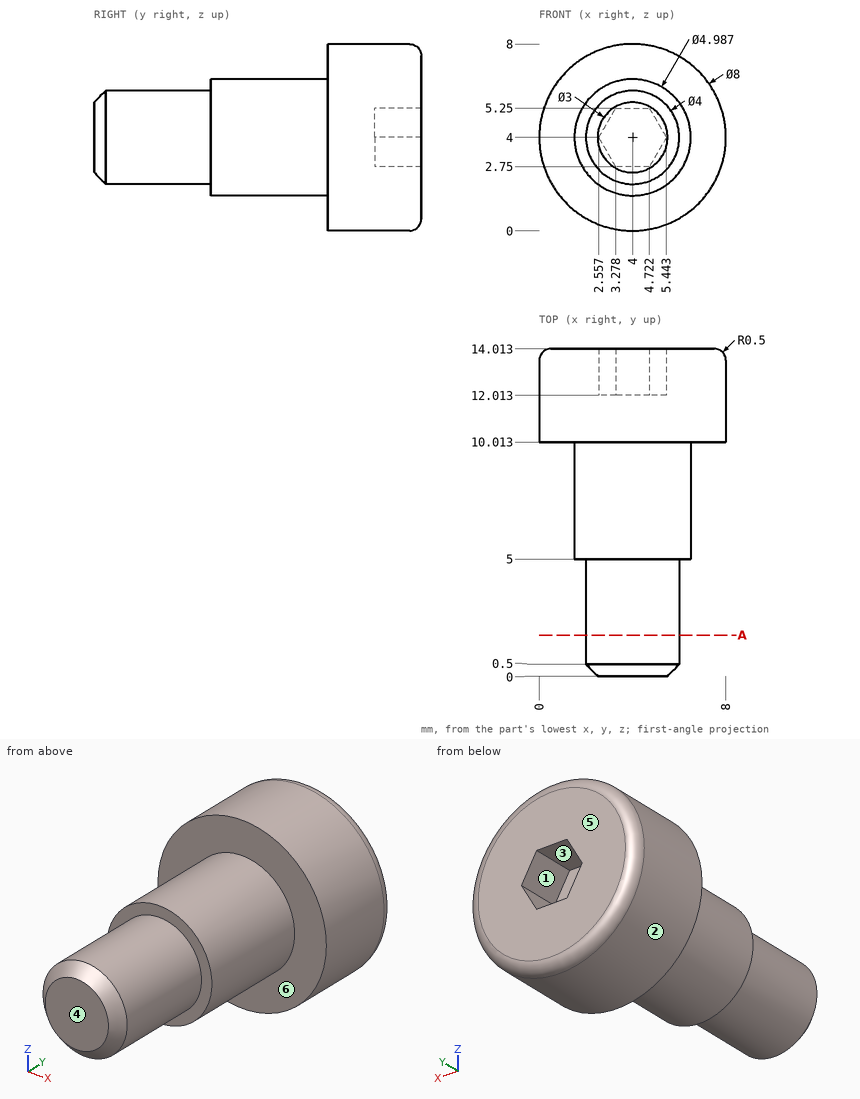
Study the drawing (mm; zero at the part's minimum x, y, z) and answer. A direction names the side the tool comes from. Coordinates: 2 decimals unless noted, no trailing zeros. Loops run counter-clockwise (first coordinate to the right, second up) from the corner with the lowest first, then second, coordinate; pieces in that order, holes last. Notation, with made-up numbers: (-6.75, -23) -> (15.25, -23) arc R26 ccw to (15.25, 13) -> close; hole circle Ø4 at (57.25, 29.5). An arc over 180 degrees is marked (long way). Write item = value, one per line. Start each with the question number.
1) The mould has two halves that part along X. Classify the marked faces 1, 2, 3 and 4: pulls with the +X half, pulls with the -X half, needs draft (parallel to the pull), parting line crosses it, or undercut.
2) Given P1, Ø1.5, axis at y = 9.5, z = 5.5, coming from the -X side (1 decimal); P2, Ø1, axis at x = 6.5, z = 2.5, coming from the -Y side; P3, Ø2, axis at x = 4.5, z = 6.5, coming from the -Y side, each flat-ended and moving along its own axis, determine where each tip first touches the part or whether it passes through.
3) Find the intervals of material crossed by L1, parallel to Y at x = 4.5, z = 3; L2, parallel to Y at x = 1.5, z = 4.75; L3, parallel to Z at x = 5.25, y = 10.5, in increasing order. Write a range as from..to.
4) For the marked faces 5 and 6, determine the directions among +Z, -Z, +X, -X, +Y, -Y from which every point of the face is accessible in a straight line to the end or side of a thin tool.
5) The part is cut by section A-A, the plane y = 1.75. Determine the outline of the cut face in (x, z), plus the area to 3 significant figures.
Result:
q1.face_1 = undercut
q1.face_2 = parting line crosses it
q1.face_3 = undercut
q1.face_4 = needs draft
q2.P1 = 0.1
q2.P2 = 5
q2.P3 = 0.05
q3.L1 = 0..12.01
q3.L2 = 10.01..14.01
q3.L3 = 0.2..7.8
q4.face_5 = +Z, -Z, +X, -X, +Y
q4.face_6 = -Y
q5.outline = circle Ø4 at (4, 4)
q5.area = 12.6 mm²
